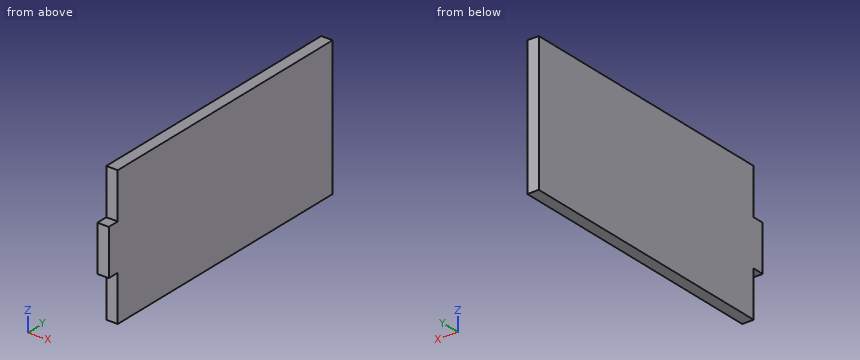
```python
from build123d import *

# Parameters (mm, degrees)
F0_W     = 3.175
F0_H     = 12.7
F1_DEPTH = 3.175


with BuildPart() as f1:
    # F0 (on Right) → F1 (new body)
    with BuildSketch(Plane.YZ):
        with Locations((-77.7875, 19.05)):
            Rectangle(F0_W, F0_H)
        Polygon((0, 0), (0, 38.1), (-76.2, 38.1), (-76.2, 25.4), (-76.2, 12.7), (-76.2, 0), align=None)
    extrude(amount=F1_DEPTH)


solid = f1.part
```
Build history of the part. All positions in model axes, mm. Round coordinates to 2 decimals unless told otherwise and drop trailing zeros. Loops run counter-clockwise (first coordinate to the right, second up) from the corner with the lowest first, then second, coordinate; pieces in that order, holes last. Notation, with made-up numbers: M 85.25,51.25 L 93.25,51.25 A14 cw 93.25,64.25 Z; hole C 42.25,55.5 d5. An arc over 180 degrees is marked long. Answer as CSV lines item,"result".
1. Cut at A-A on x = 1.3. Write the cut outline in (y, z) (3 decimals), then the cut area to 3 significant figures.
Resolved:
outline,"M -79.375,12.7 L -76.2,12.7 L -76.2,0 L 0,0 L 0,38.1 L -76.2,38.1 L -76.2,25.4 L -79.375,25.4 Z"
area,"2,940 mm²"
2. Cut at B-B on z = 11. Write the cut outline in (x, y) (3 decimals), then the cut area to 3 significant figures.
Resolved:
outline,"M 0,-76.2 L 3.175,-76.2 L 3.175,0 L 0,0 Z"
area,"242 mm²"
3. Wall check: probe 1 along Y at (x, z) = (1.3, 31). Give the ranges that are in metal, low to high. Write a range as [from, to].
Resolved:
probe 1,"y = [-76.2, 0]"
